Design review of the part built by this model. Coordinates are the model's own, in mm. Round coordinates to 2 decimals unless told otherwise and drop trailing zeros. Loops run counter-clockwise (first coordinate to the right, second up) from the corner with the lowest first, then second, coordinate; pieces in that order, holes last. Notation, with made-up numbers: M 85.25,31.25 L 112.25,31.25 A21 cw 112.25,39.25 Z; hole C 78,51 d1. An arc over 180 degrees is marked long. One line per item, written item: value. Start each with the question number.
Item 1: For line 1 along Z through (x, y) = (12, -74.25); line 2 along Z through (x, y) = (16, -74); line 3 along Y through (x, z) = (25, 3.25), list the stretches that pass through material, from the lowest coordinate up.
Item 2: We need section A-A (x = 0). Write out the cut boundary in (y, z), then the cut area to 3 significant figures.
Item 3: Clearance check with a flat-ended pin moving along its axis: pin 1 (2 mm diameter, centred on x = 24, z = 2.9, fed in from -Y). State where the tip first meets the part, or that it passes through.
from build123d import *

# Parameters (mm, degrees)
CYLINDER005_R     = 1.2
CYLINDER005_DEPTH = 1.8
ARRAY007_X_COUNT  = 7
ARRAY007_X_PITCH  = 4
BOX015_W          = 64
BOX015_H          = 10
BOX015_DEPTH      = 13.2
FILLET006_R       = 2


with BuildPart() as array007:
    # Cylinder005 → Cylinder005 (new body)
    with BuildSketch(Plane(origin=(0, -73.5, 2.9), x_dir=(1, 0, 0), z_dir=(0, -1, 0))):
        Circle(CYLINDER005_R)
    extrude(amount=CYLINDER005_DEPTH)

    # Array007 X: Array007 ×7


with BuildPart() as array007_1:
    add(array007.part)
    with Locations(*[(i * ARRAY007_X_PITCH, 0, 0) for i in range(1, ARRAY007_X_COUNT)]):
        add(array007.part)


with BuildPart() as seitenteil:
    # Box015 → Box015 (new body)
    with BuildSketch(Plane(origin=(-32, -75, -1.4), x_dir=(1, 0, 0), z_dir=(0, 0, 1))):
        with Locations((32, 5)):
            Rectangle(BOX015_W, BOX015_H)
    extrude(amount=BOX015_DEPTH)

    # Fillet006
    fillet006_edges = [seitenteil.edges().sort_by_distance(p)[0] for p in [
        (-32, -75, 5.2),
        (-32, -70, 11.8),
        (-32, -65, 5.2),
        (32, -75, 5.2),
        (32, -70, 11.8),
        (32, -65, 5.2),
        (0, -75, 11.8),
        (0, -65, 11.8),
    ]]
    fillet(fillet006_edges, radius=FILLET006_R)

    # Cut010: cut Array007
    add(array007_1.part, mode=Mode.SUBTRACT)


solid = seitenteil.part
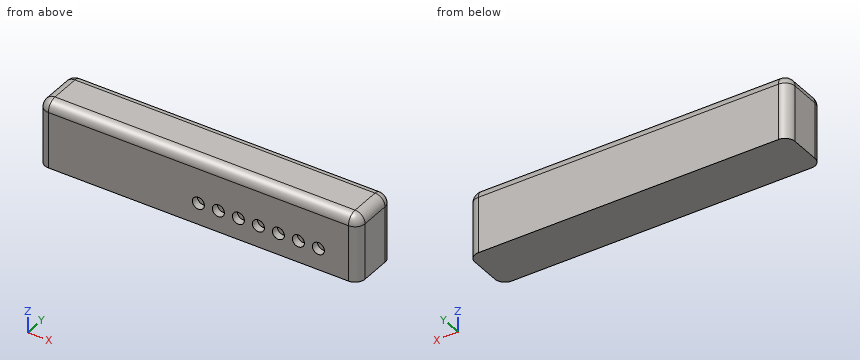
A:
1. line 1: -1.4 to 1.7, 4.1 to 11.36
1. line 2: -1.4 to 1.7, 4.1 to 11.53
1. line 3: -73.5 to -65
2. outline: M -75,-1.4 L -65,-1.4 L -65,9.8 A2 ccw -67,11.8 L -73,11.8 A2 ccw -75,9.8 L -75,4.1 L -73.5,4.1 L -73.5,1.7 L -75,1.7 Z
2. area: 127 mm2
3. pin 1: y = -73.5
